from build123d import *

# Parameters (mm, degrees)
BOSS_EXTRUDE4_DEPTH     = 10
CUT_EXTRUDE2_DEPTH      = 39.890872965
CUT_EXTRUDE2_DEPTH_BACK = 39.890872965
CUT_EXTRUDE3_REACH      = 57
SKETCH7_R               = 3
CUT_EXTRUDE4_REACH      = 57
SKETCH8_R               = 3
CUT_EXTRUDE5_REACH      = 29.5
SKETCH9_R               = 1


with BuildPart() as part:
    # Sketch4 → Boss-Extrude4 (new body)
    with BuildSketch(Plane.XY):
        Polygon((38.890872965, -10), (0, 28.890872965), (-38.890872965, -10), align=None)
        Polygon((0, 21.819805153), (21.819805153, 0), (14.748737342, 0), (-14.748737342, 0), (-21.819805153, 0), align=None, mode=Mode.SUBTRACT)
    extrude(amount=BOSS_EXTRUDE4_DEPTH)

    # Sketch6 → Cut-Extrude2 (cut, two sides)
    with BuildSketch(Plane(origin=(0, 0, 0), x_dir=(0, 0, -1), z_dir=(1, 0, 0))) as cut_extrude2_sk:
        Polygon((-10, -10), (0, 0), (0, -10), align=None)
    extrude(amount=CUT_EXTRUDE2_DEPTH, mode=Mode.SUBTRACT)
    extrude(cut_extrude2_sk.sketch, amount=-CUT_EXTRUDE2_DEPTH_BACK, mode=Mode.SUBTRACT)

    # Sketch7 → Cut-Extrude3 (cut, up to next)
    with BuildSketch(Plane(origin=(-14.445436483, 14.445436483, 0), x_dir=(0, 0, 1), z_dir=(-0.707106781, 0.707106781, 0)), mode=Mode.PRIVATE) as cut_extrude3_sk1:
        with Locations((5, -9.571067812)):
            Circle(SKETCH7_R)
    cut_extrude3_tool1 = extrude(cut_extrude3_sk1.sketch, amount=-CUT_EXTRUDE3_REACH, mode=Mode.PRIVATE) & part.part
    add(cut_extrude3_tool1.solids().sort_by_distance((-21.213203, 7.67767, 5))[0], mode=Mode.SUBTRACT)

    # Sketch8 → Cut-Extrude4 (cut, up to next)
    with BuildSketch(Plane(origin=(14.445436483, 14.445436483, 0), x_dir=(0, 0, -1), z_dir=(0.707106781, 0.707106781, 0)), mode=Mode.PRIVATE) as cut_extrude4_sk1:
        with Locations((-5, -9.571067812)):
            Circle(SKETCH8_R)
    cut_extrude4_tool1 = extrude(cut_extrude4_sk1.sketch, amount=-CUT_EXTRUDE4_REACH, mode=Mode.PRIVATE) & part.part
    add(cut_extrude4_tool1.solids().sort_by_distance((21.213203, 7.67767, 5))[0], mode=Mode.SUBTRACT)

    # Sketch9 → Cut-Extrude5 (cut, up to next)
    with BuildSketch(Plane(origin=(0, 0, 0), x_dir=(1, 0, 0), z_dir=(0, -0.707106781, -0.707106781)), mode=Mode.PRIVATE) as cut_extrude5_sk1:
        with Locations((-14, 7)):
            Circle(SKETCH9_R)
    cut_extrude5_tool1 = extrude(cut_extrude5_sk1.sketch, amount=-CUT_EXTRUDE5_REACH, mode=Mode.PRIVATE) & part.part
    add(cut_extrude5_tool1.solids().sort_by_distance((-14, -4.949747, 4.949747))[0], mode=Mode.SUBTRACT)
    # Sketch9 → Cut-Extrude5 (cut, up to next)
    with BuildSketch(Plane(origin=(0, 0, 0), x_dir=(1, 0, 0), z_dir=(0, -0.707106781, -0.707106781)), mode=Mode.PRIVATE) as cut_extrude5_sk2:
        with Locations((14, 7)):
            Circle(SKETCH9_R)
    cut_extrude5_tool2 = extrude(cut_extrude5_sk2.sketch, amount=-CUT_EXTRUDE5_REACH, mode=Mode.PRIVATE) & part.part
    add(cut_extrude5_tool2.solids().sort_by_distance((14, -4.949747, 4.949747))[0], mode=Mode.SUBTRACT)


solid = part.part
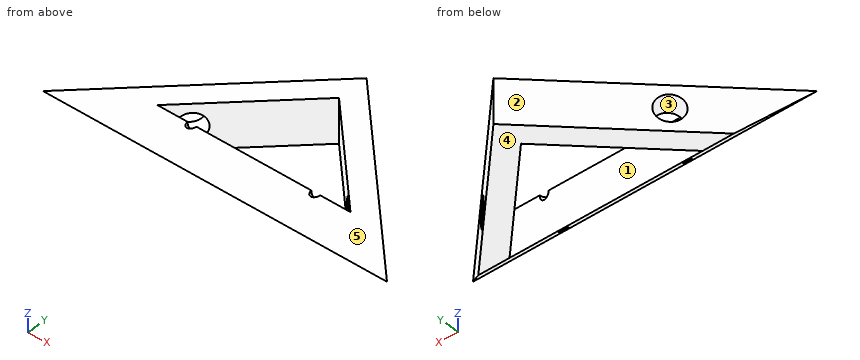
Design review of the part built by this model. Coordinates are the model's own, in mm. Face numbers are marked on the shaded views. A direction names the side the tool comes from. Coordinates: 2 decimals unless noted, no trailing zeros. Loops run counter-clockwise (first coordinate to the right, second up) from the corner with the lowest first, then second, coordinate; pieces in that order, holes last. Notation, with made-up numbers: (66.25, 47) -> (73.25, 47) arc R17 ccw to (73.25, 80) -> close; hole circle Ø2 at (1, 52.25). An arc over 180 degrees is marked (long way). Use a Markdown table: item, result. Add a question column.
Item 1: We need section A-A, the plane y = 15.5. Write out the cut boundary in (x, z), and give its area (3 significant figures).
Item 2: Wall thickness on L1, parallel to X at y = -1.5, z = 8; L2, parallel to Z at x = -14, y = -4; L3, parallel to X at y = 14, z = 7.5: over which ranges is each line inside the solid? List them lowest first. Write a range as from..to.
Item 3: Clearance check with flat-ended pins moving along their axes: P1, Ø4, axis at x = -8, z = 7, coming from the +Y side; P2, Ø5, axis at y = 17, z = 4.5, coming from the +X side; P3, Ø12, axis at x = -27, y = 8.5, coming from the -Z side; P4, Ø6, axis at y = 23.5, z = 6, coming from the +X side. State where each tip first meets the part, or that it passes through.
Item 4: We need section B-B, the plane z = 6. Count the separate pieces of the cut face and the enclosed holes in it, and give its area (3 significant figures).
Item 5: Machinability: for the marked faces 1 and 2, which of the approach directions +Z, -Z, +X, -X, +Y, -Y give a long, thin tool a straight path to every point of the face, cutting with its end or side? Answer none if there is none.
Item 6: We need section C-C, the plane x = 32.5. Write out the cut boundary in (y, z), and give its area (3 significant figures).
Item 7: The part is to be moulded in two halves that separate along Z. For the marked faces 3, 4 and 5, say which applies: +Z half, -Z half, draft (parallel to the pull), parting line (faces both ways), or undercut.
Numbers:
| question | item | result |
|---|---|---|
| 1 | outline | (-13.39, 0) -> (-6.32, 0) -> (-6.32, 10) -> (-13.39, 10) -> close; (6.32, 0) -> (13.39, 0) -> (13.39, 10) -> (6.32, 10) -> close |
| 1 | area | 141 mm^2 |
| 2 | L1 | x = -30.39..-14.96, -13.04..13.04, 14.96..30.39 |
| 2 | L2 | z = 4..4.49, 7.31..10 |
| 2 | L3 | x = -14.89..-7.82, 7.82..14.89 |
| 3 | P1 | stops at y = 22.89 |
| 3 | P2 | stops at x = 14.39 |
| 3 | P3 | stops at z = 0 |
| 3 | P4 | stops at x = 8.39 |
| 4 | separate pieces | 2 |
| 4 | enclosed holes | 2 |
| 4 | area | 676 mm^2 |
| 5 | face 1 | +Z, -Z |
| 5 | face 2 | +Z, -Z, -X, +Y |
| 6 | outline | (-10, 10) -> (-3.61, 3.61) -> (-3.61, 10) -> close |
| 6 | area | 20.4 mm^2 |
| 7 | face 3 | undercut |
| 7 | face 4 | -Z half |
| 7 | face 5 | +Z half |
